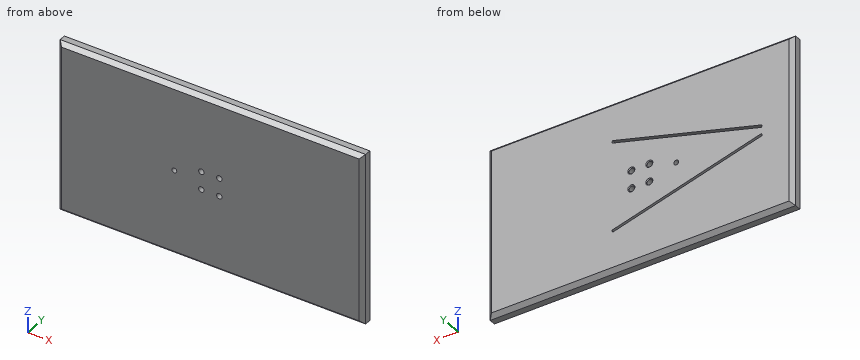
Autodesk Inventor part; units mm, degrees
ref_plane "YZ Plane" through (0, 0, 0) normal (1, 0, 0) x (0, 1, 0)
ref_plane "XZ Plane" through (0, 0, 0) normal (0, 1, 0) x (-1, 0, 0)
ref_plane "XY Plane" through (0, 0, 0) normal (0, 0, 1) x (1, 0, 0)
sketch "Sketch1" plane through (0, 0, 0) normal (0, 1, 0) x (-1, 0, 0)
  line L0 (0, 0) -> (390, 0)
  line L1 (390, 0) -> (390, -219)
  line L2 (390, -219) -> (0, -219)
  line L3 (0, -219) -> (0, 0)
  dimension "d0" = 219
  dimension "d1" = 390
extrude "Platform" add sketch "Sketch1" along normal blind 18
sketch "Sketch3" plane through (0, 18, 0) normal (0, 1, 0) x (1, 0, 0)
  circle A0 centre (-240.9586, 109.5) radius 3.1
  line L0 (0, 0) -> (0, 219)
  line L1 (-390, 0) -> (0, 0)
  line L2 (-229.5, 144) -> (-160.5, 144)
  line L3 (-160.5, 144) -> (-160.5, 75)
  line L4 (-160.5, 75) -> (-229.5, 75)
  line L5 (-229.5, 75) -> (-229.5, 144)
  line L6 (-206.5, 121) -> (-183.5, 98)
  circle A1 centre (-206.5, 121) radius 3.5
  circle A2 centre (-183.5, 98) radius 3.5
  circle A3 centre (-183.5, 121) radius 3.5
  circle A4 centre (-206.5, 98) radius 3.5
  line L7 (-206.5, 98) -> (-183.5, 121)
  point P0 (0, 109.5)
  point P1 (-195, 109.5)
  point P2 (-160.5, 109.5)
  point P3 (-195, 144)
  point P4 (0, 109.5)
  point P5 (-195, 0)
  dimension "screwdiameter" = 6.2
  dimension "d34" = 69
  dimension "d35" = 69
  dimension "d36" = 7
  dimension "d37" = 7
  dimension "d38" = 7
  dimension "d39" = 7
  dimension "d43" = 23
extrude "ScrewHole" cut sketch "Sketch3" against normal through all contours A0 | A3 | A2 | A4 | A1
sketch "Sketch2" plane through (0, 18, 0) normal (0, 1, 0) x (1, 0, 0)
  line L0 (-364.182, 109.5) -> (-365, 112.4901)
  line L1 (-365, 112.4901) -> (-145.0809, 172.6532)
  line L2 (-145.0809, 172.6532) -> (-144.2629, 169.6631)
  line L3 (-144.2629, 169.6631) -> (-364.182, 109.5)
  line L4 (0, 0) -> (0, 219)
  line L5 (18.6218, 109.5) -> (45.6135, 109.5)
  line L6 (-390, 0) -> (0, 0)
  line L7 (-364.182, 109.5) -> (-365, 106.5099)
  line L8 (-365, 106.5099) -> (-145.0809, 46.3468)
  line L9 (-145.0809, 46.3468) -> (-144.2629, 49.3369)
  line L10 (-144.2629, 49.3369) -> (-364.182, 109.5)
  line L11 (-350.5799, 116.435) -> (-349.7619, 113.4449)
  line L12 (-159.501, 168.7083) -> (-158.683, 165.7182)
  line L13 (-350.5799, 102.565) -> (-349.7619, 105.5551)
  line L14 (-159.501, 50.2917) -> (-158.683, 53.2818)
  line L15 (-390, 219) -> (-390, 0)
  point P0 (32.1177, 109.5)
  point P1 (0, 109.5)
  point P2 (-195, 0)
  point P3 (-254.2224, 139.5815)
  point P4 (-159.501, 50.2917)
  point P5 (-158.683, 53.2818)
  point P6 (-350.5799, 102.565)
  dimension "d6" = 3.1
  dimension "beta" = 15.3
  dimension "rail" = 228
  dimension "centre_offset" = 0
  dimension "offsetlength" = 14.95
  dimension "d20" = 14.95
  dimension "d44" = 198.1
  dimension "d52" = 25
extrude "Slots" cut sketch "Sketch2" against normal blind 5 contours L11 L1 L12 L3 | L10 L14 L8 L13
chamfer "Chamfer1" distance 5 angle 45 8 edges at (-390, 18, -109.5) (-195, 18, 0) (-195, 18, -219) (0, 18, -109.5) (0, 0, -109.5) (-195, 0, 0) (-390, 0, -109.5) (-195, 0, -219)
chamfer "Countersunk" distance 1 angle 45 4 edges at (-210, 18, -98) (-210, 18, -121) (-187, 18, -121) (-187, 18, -98)
sketch "InstructionsSticker" plane through (0, 18, 0) normal (0, 1, 0) x (1, 0, 0)
  line L0 (-120, 15) -> (-15, 15)
  line L1 (-15, 15) -> (-15, 204)
  line L2 (-15, 204) -> (-120, 204)
  line L3 (-120, 204) -> (-120, 15)
  line L4 (0, 219) -> (-390, 219)
  line L5 (-390, 0) -> (0, 0)
  line L6 (0, 0) -> (0, 219)
  line L7 (-120, 204) -> (-15.0037, 204) construction
  line L8 (-15.0037, 204) -> (-15.0037, 14.9979) construction
  line L9 (-15.0037, 14.9979) -> (-120, 14.9979) construction
  line L10 (-120, 14.9979) -> (-120, 204) construction
  dimension "d53" = 105
  dimension "d54" = 15
  dimension "d55" = 15
  dimension "d56" = 15
  dimension "d58" = 189
equation "\"d20\" = offsetlength"
equation "\"gluegap\" = 0.1"
properties part number "platform_instr"
The listing builds one solid part. Answer for the finished solid, in the listing's coordinates (mm). Give positions to 0.01 mm unless a question says otherwise; leave off trailing zeros. Loops run counter-clockwise (first coordinate to the right, second up) from the corner with the lowest first, then second, coordinate; pieces in that order, holes last. Notation, with made-up numbers: (52, -13) - (84, -13) arc R18 cw to (84, 18) - close; hole circle Ø9 at (-16.75, 56.5). An arc over 180 degrees is marked (long way). Write each question's results on one line, items separated by ' | '.
1. Find section A-A, the plane z = -62. Write down the section's boundary in (x, y).
Resolved:
outline: (-390, 5) - (-385, 0) - (-5, 0) - (0, 5) - (0, 13) - (-5, 18) - (-190.55, 18) - (-190.55, 13) - (-202.3, 13) - (-202.3, 18) - (-385, 18) - (-390, 13) - close
2. Consider probe 1 along Z at (x, y) = (-183.5, 12.25); probe 2 along X at (y, z) = (12.5, -121); probe 3 along X at (y, z) = (4.5, -121). Determine where each line is inside the solid, lowest interval first. Write a range as from..to.
Resolved:
probe 1: z = -219..-124.5, -117.5..-101.5, -94.5..0 | probe 2: x = -390..-210, -203..-187, -180..0 | probe 3: x = -389.5..-210, -203..-187, -180..-0.5
3. Flat-ended cylindrical pins translate along their axes: P1, Ø8, axis at x = -68.5, y = 4.5, coming from the +Z side; P2, Ø4, axis at x = -206.5, z = -121, coming from the -Y side. Find the tip coordinate at first contact, or state that the pin passes through.
Resolved:
P1: stops at z = 0 | P2: passes through
4. Find section B-B, the plane x = -310. Write down the section's boundary in (y, z).
Resolved:
outline: (0, -214) - (5, -219) - (13, -219) - (18, -214) - (18, -127.54) - (13, -127.54) - (13, -124.32) - (18, -124.32) - (18, -94.68) - (13, -94.68) - (13, -91.46) - (18, -91.46) - (18, -5) - (13, 0) - (5, 0) - (0, -5) - close
